Could you check a few things on this model? Use its own coordinates, in mm. A direction names the side the tool comes from. Give positions to 0.01 mm unless a question says otherwise; leave off trailing zeros. Loops run counter-clockwise (first coordinate to the right, second up) from the corner with the lowest first, then second, coordinate; pieces in that order, holes last.
1. I need wall thicknesses on line 1 along Z through (x, y) = (-50.8, -2.55); line 2 along X through (y, z) = (69, 25); line 3 along Z through (x, y) = (-10, 49). Which ranges of each line are inside material? Lowest first, please.
2. Imagine slicing it at B-B (z = 0). Count the separate pieces of the cut face and the enclosed holes in it, plus the area to 3 significant figures.
3. For P1, Ø4, axis at x = 20, y = 60.5, coming from the -Z side; P2, Ø9, axis at x = -76.2, z = -68.26, coming from the +Y side; P3, Ø1, axis at x = -65, y = 20.5, coming from the +Z side, each with a flat end and sliding along its axis, tell me the tip position at first contact or that it passes through.
4. Thinking about a two-plate mould opening in Z: for faces 4 (the flat face through (-39, 74.676, 1)), 5 (the flat face through (-39, -3, -77.66)), 6 (the cylindrical face through (-88.63, 76.25, -7.94)), which applies, +Z half, -Z half, draft (parallel to the pull), parting line (faces both ways), or undercut?
5. Imagine slicing it at A-A (y = 13.5). List the corners of the cut face in (x, z) for me.
6. For faces 1 (the flat face through (-39, 0, -67)), 2 (the flat face through (-119.15, 28, -1)), 3 (the flat face through (6, 65.024, 17)), which set-ups out of +Z, -Z, +X, -X, +Y, -Y let a thin tool reach every point of the face, with its end or its side?
```python
from build123d import *

# Parameters (mm, degrees)
BOSS_EXTRUDE1_DEPTH        = 44.45
BOSS_EXTRUDE1_DEPTH_BACK   = 120.65
SKETCH5_W                  = 99.125
SKETCH5_H                  = 72.176
BOSS_EXTRUDE2_DEPTH        = 1.5
CUT_EXTRUDE1_DEPTH         = 101.6
SKETCH12_R                 = 29
BOSS_EXTRUDE3_DEPTH        = 4.1
CHAMFER1_SIZE              = 4.1
SKETCH10_R                 = 2.05
CUT_EXTRUDE2_DEPTH         = 164.686388977
BOSS_EXTRUDE4_START        = -8.5
SKETCH17_R                 = 19.05
BOSS_EXTRUDE4_DEPTH        = 9.652
SKETCH13_R                 = 17.4625
CUT_EXTRUDE4_DEPTH         = 164.686388977
CHAMFER3_SIZE              = 1
LPATTERN1_COUNT            = 2
LPATTERN1_PITCH            = 82.55
CHAMFER1_OF_LPATTERN1_SIZE = 4.1
SKETCH14_R                 = 5
CUT_EXTRUDE5_DEPTH         = 164.686388977
SKETCH15_R                 = 10
CUT_EXTRUDE6_DEPTH         = 4.1
FILLET1_R                  = 1.27
FILLET3_R                  = 5
CHAMFER4_SIZE              = 1
CHAMFER5_SIZE              = 3
CHAMFER5_SIZE2             = 2.517298894


# Some blends are built 0.0001 mm under size
with BuildPart() as part:
    # Sketch2 → Boss-Extrude1 (new, two sides: drawn at the far end of the back side and taken through both)
    with BuildSketch(Plane(origin=(0, 0, 0), x_dir=(0, 0, -1), z_dir=(1, 0, 0)).offset(-BOSS_EXTRUDE1_DEPTH_BACK)):
        Polygon((-77.6605, 0), (-55.5625, 0), (-55.5625, 74.676), (55.5625, 74.676), (55.5625, 0), (77.6605, 0), (77.6605, -6), (49.5625, -6), (49.5625, 66.176), (-49.5625, 66.176), (-49.5625, -6), (-77.6605, -6), align=None)
    extrude(amount=BOSS_EXTRUDE1_DEPTH + BOSS_EXTRUDE1_DEPTH_BACK)

    # Sketch5 → Boss-Extrude2 (add)
    with BuildSketch(Plane.ZY.offset(120.65)):
        with Locations((0, 30.088)):
            Rectangle(SKETCH5_W, SKETCH5_H)
    extrude(amount=-BOSS_EXTRUDE2_DEPTH)

    # Sketch4 → Cut-Extrude1 (cut)
    with BuildSketch(Plane(origin=(0, 0, 0), x_dir=(1, 0, 0), z_dir=(0, 1, 0))):
        with BuildLine():
            Line((-98.85, 68.2625), (-98.85, 71.4375))
            ThreePointArc((-98.85, 71.4375), (-102.432865533, 74.058346238), (-103.845516366, 69.85))
            ThreePointArc((-103.845516366, 69.85), (-102.432865533, 65.641653762), (-98.85, 68.2625))
        make_face()
        with BuildLine():
            Line((-73.45, 68.2625), (-73.45, 71.4375))
            ThreePointArc((-73.45, 71.4375), (-77.032865533, 74.058346238), (-78.445516366, 69.85))
            ThreePointArc((-78.445516366, 69.85), (-77.032865533, 65.641653762), (-73.45, 68.2625))
        make_face()
        with BuildLine():
            Line((-48.05, 68.2625), (-48.05, 71.4375))
            ThreePointArc((-48.05, 71.4375), (-51.632865533, 74.058346238), (-53.045516366, 69.85))
            ThreePointArc((-53.045516366, 69.85), (-51.632865533, 65.641653762), (-48.05, 68.2625))
        make_face()
        with BuildLine():
            Line((-22.65, 68.2625), (-22.65, 71.4375))
            ThreePointArc((-22.65, 71.4375), (-26.232865533, 74.058346238), (-27.645516366, 69.85))
            ThreePointArc((-27.645516366, 69.85), (-26.232865533, 65.641653762), (-22.65, 68.2625))
        make_face()
        with BuildLine():
            Line((2.75, 68.2625), (2.75, 71.4375))
            ThreePointArc((2.75, 71.4375), (-0.832865533, 74.058346238), (-2.245516366, 69.85))
            ThreePointArc((-2.245516366, 69.85), (-0.832865533, 65.641653762), (2.75, 68.2625))
        make_face()
        with BuildLine():
            Line((28.15, 68.2625), (28.15, 71.4375))
            ThreePointArc((28.15, 71.4375), (24.567134467, 74.058346238), (23.154483634, 69.85))
            ThreePointArc((23.154483634, 69.85), (24.567134467, 65.641653762), (28.15, 68.2625))
        make_face()
    cut_extrude1 = extrude(amount=-CUT_EXTRUDE1_DEPTH, mode=Mode.SUBTRACT)

    # Mirror1: Cut-Extrude1 across plane
    add(cut_extrude1.mirror(Plane.XY), mode=Mode.SUBTRACT)

    # Sketch12 → Boss-Extrude3 (add)
    with BuildSketch(Plane(origin=(0, 74.676, 0), x_dir=(1, 0, 0), z_dir=(0, 1, 0))):
        with Locations(Location((0, 0, 0), (0, 0, 270))):
            Circle(SKETCH12_R)
    boss_extrude3 = extrude(amount=BOSS_EXTRUDE3_DEPTH)

    # Chamfer1
    chamfer1_edges = [part.edges().sort_by_distance(p)[0] for p in [
        (0, 74.676, -29),
    ]]
    chamfer(chamfer1_edges, length=CHAMFER1_SIZE - 0.0001)  # a hair under: the kernel refuses the full size

    # Sketch10 → Cut-Extrude2 (cut, symmetric)
    with BuildSketch(Plane(origin=(0, 0, 0), x_dir=(1, 0, 0), z_dir=(0, 1, 0))):
        with Locations(Location((17.960512242, 17.960512242, 0), (0, 0, 270))):
            Circle(SKETCH10_R)
        with Locations(Location((25.4, 0, 0), (0, 0, 270))):
            Circle(SKETCH10_R)
        with Locations(Location((17.960512242, -17.960512242, 0), (0, 0, 270))):
            Circle(SKETCH10_R)
        with Locations(Location((0, -25.4, 0), (0, 0, 270))):
            Circle(SKETCH10_R)
        with Locations(Location((-17.960512242, -17.960512242, 0), (0, 0, 270))):
            Circle(SKETCH10_R)
        with Locations(Location((-25.4, 0, 0), (0, 0, 270))):
            Circle(SKETCH10_R)
        with Locations(Location((-17.960512242, 17.960512242, 0), (0, 0, 270))):
            Circle(SKETCH10_R)
        with Locations(Location((0, 25.4, 0), (0, 0, 270))):
            Circle(SKETCH10_R)
    cut_extrude2 = extrude(amount=CUT_EXTRUDE2_DEPTH, both=True, mode=Mode.SUBTRACT)

    # Sketch17 → Boss-Extrude4 (add)
    with BuildSketch(Plane.XZ.offset(-66.176).offset(BOSS_EXTRUDE4_START)):
        with Locations(Location((0, 0, 0), (0, 0, 90))):
            Circle(SKETCH17_R)
    extrude(amount=BOSS_EXTRUDE4_DEPTH)

    # Sketch13 → Cut-Extrude4 (cut, through all)
    with BuildSketch(Plane(origin=(0, 0, 0), x_dir=(1, 0, 0), z_dir=(0, 1, 0))):
        with Locations(Location((0, 0, 0), (0, 0, 90))):
            Circle(SKETCH13_R)
    extrude(amount=CUT_EXTRUDE4_DEPTH, mode=Mode.SUBTRACT)

    # Chamfer3
    chamfer3_edges = [part.edges().sort_by_distance(p)[0] for p in [
        (0, 66.176, -19.05),
    ]]
    chamfer(chamfer3_edges, length=CHAMFER3_SIZE)

    # LPattern1: Boss-Extrude3, Cut-Extrude2 ×2
    with Locations(*[(-i * LPATTERN1_PITCH, 0, 0) for i in range(1, LPATTERN1_COUNT)]):
        add(boss_extrude3)
        add(cut_extrude2, mode=Mode.SUBTRACT)

    # Chamfer1 of LPattern1
    chamfer1_of_lpattern1_edges = [part.edges().sort_by_distance(p)[0] for p in [
        (-82.55, 74.676, -29),
    ]]
    chamfer(chamfer1_of_lpattern1_edges, length=CHAMFER1_OF_LPATTERN1_SIZE - 0.0001)  # a hair under: the kernel refuses the full size

    # Sketch14 → Cut-Extrude5 (cut, through all)
    with BuildSketch(Plane(origin=(0, 0, 0), x_dir=(1, 0, 0), z_dir=(0, 1, 0))):
        with Locations(Location((-82.55, 0, 0), (0, 0, 270))):
            Circle(SKETCH14_R)
    extrude(amount=CUT_EXTRUDE5_DEPTH, mode=Mode.SUBTRACT)

    # Sketch15 → Cut-Extrude6 (cut)
    with BuildSketch(Plane(origin=(0, 78.776, 0), x_dir=(1, 0, 0), z_dir=(0, 1, 0))):
        with Locations(Location((-82.55, 0, 0), (0, 0, 270))):
            Circle(SKETCH15_R)
    extrude(amount=-CUT_EXTRUDE6_DEPTH, mode=Mode.SUBTRACT)

    # Fillet1
    fillet1_edges = [part.edges().sort_by_distance(p)[0] for p in [
        (-38.1, 0, -55.5625),
        (-38.1, 74.676, -55.5625),
        (-38.1, 74.676, 55.5625),
        (-38.1, 0, 55.5625),
        (-37.35, -6, 49.5625),
        (-37.35, -6, -49.5625),
    ]]
    fillet(fillet1_edges, radius=FILLET1_R)

    # Fillet3
    # the kernel refuses this fillet: 5 mm, written as the material it adds along each edge
    with BuildSketch(Plane(origin=(-114.15, 61.176, 44.5625), x_dir=(0, 1, 0), z_dir=(-1, 0, 0))) as fillet3_piece_1_section:
        Polygon((0, 0), (FILLET3_R * 1.02, 0), (FILLET3_R * 1.02, -FILLET3_R * 1.02), (0, -FILLET3_R * 1.02), align=None)
    fillet3_piece_1 = extrude(amount=FILLET3_R * 1.02, mode=Mode.PRIVATE)
    fillet3_piece_1 = fillet3_piece_1 - Plane(origin=(-114.15, 61.176, 44.5625), x_dir=(0, -0.7071067811865475, -0.7071067811865475), z_dir=(-1, 0, 0)) * Sphere(FILLET3_R, mode=Mode.PRIVATE)
    add(fillet3_piece_1)
    with BuildSketch(Plane(origin=(-114.15, 61.176, -44.5625), x_dir=(-1, 0, 0), z_dir=(0, 1, 0))) as fillet3_piece_2_section:
        Polygon((0, 0), (FILLET3_R * 1.02, 0), (FILLET3_R * 1.02, -FILLET3_R * 1.02), (0, -FILLET3_R * 1.02), align=None)
    fillet3_piece_2 = extrude(amount=FILLET3_R * 1.02, mode=Mode.PRIVATE)
    fillet3_piece_2 = fillet3_piece_2 - Plane(origin=(-114.15, 61.176, -44.5625), x_dir=(0.7071067811865475, 0, 0.7071067811865475), z_dir=(0, 1, 0)) * Sphere(FILLET3_R, mode=Mode.PRIVATE)
    add(fillet3_piece_2)
    with BuildSketch(Plane(origin=(-119.15, -4.73, 49.5625), x_dir=(1, 0, 0), z_dir=(0, 1, 0))) as fillet3_piece_3:
        with BuildLine():
            CenterArc((FILLET3_R, FILLET3_R), FILLET3_R, 180, 90)
            Line((0, FILLET3_R), (0, 0))
            Line((0, 0), (FILLET3_R, 0))
        make_face()
    extrude(amount=65.906)
    with BuildSketch(Plane(origin=(-119.15, -4.73, -50.8325), x_dir=(0, 0.006283143965557515, 0.9999802608561371), z_dir=(0, -0.9999802608561371, 0.006283143965557515))) as fillet3_piece_4_section:
        with BuildLine():
            CenterArc((-1.27 - FILLET3_R, -FILLET3_R), FILLET3_R, 0, 90)
            Line((-1.27 - FILLET3_R, 0), (-1.27, 0))
            Line((-1.27, 0), (-1.27, -FILLET3_R))
        make_face()
    fillet3_piece_4 = revolve(axis=Axis((-119.15, -4.73, -50.8325), (-1, 0, 0)), revolution_arc=359.64, mode=Mode.PRIVATE)
    fillet3_piece_4 = split(fillet3_piece_4, bisect_by=Plane(origin=(-117.187917089, -6, -49.859640049), z_dir=(0, 1, 0)), keep=Keep.TOP, mode=Mode.PRIVATE)
    add(fillet3_piece_4)
    with BuildSketch(Plane(origin=(-119.15, -4.73, 50.8325), x_dir=(0, 0.006283143965559613, -0.9999802608561371), z_dir=(0, -0.9999802608561371, -0.006283143965559613))) as fillet3_piece_5_section:
        with BuildLine():
            CenterArc((-1.27 - FILLET3_R, FILLET3_R), FILLET3_R, 270, 90)
            Line((-1.27 - FILLET3_R, 0), (-1.27, 0))
            Line((-1.27, 0), (-1.27, FILLET3_R))
        make_face()
    fillet3_piece_5 = revolve(axis=Axis((-119.15, -4.73, 50.8325), (1, 0, 0)), revolution_arc=359.64, mode=Mode.PRIVATE)
    fillet3_piece_5 = split(fillet3_piece_5, bisect_by=Plane(origin=(-117.187917089, -6, 49.85964009), z_dir=(0, 1, 0)), keep=Keep.TOP, mode=Mode.PRIVATE)
    add(fillet3_piece_5)
    with BuildSketch(Plane(origin=(44.45, 66.176, 49.5625), x_dir=(0, 0, -1), z_dir=(-1, 0, 0))) as fillet3_piece_6:
        with BuildLine():
            CenterArc((FILLET3_R, FILLET3_R), FILLET3_R, 180, 90)
            Line((0, FILLET3_R), (0, 0))
            Line((0, 0), (FILLET3_R, 0))
        make_face()
    extrude(amount=158.6)
    with BuildSketch(Plane(origin=(44.45, 66.176, -49.5625), x_dir=(0, 0, 1), z_dir=(-1, 0, 0))) as fillet3_piece_7:
        with BuildLine():
            CenterArc((FILLET3_R, -FILLET3_R), FILLET3_R, 90, 90)
            Line((0, -FILLET3_R), (0, 0))
            Line((0, 0), (FILLET3_R, 0))
        make_face()
    extrude(amount=158.6)
    with BuildSketch(Plane(origin=(-119.15, 61.176, -49.5625), x_dir=(0, 0, 1), z_dir=(0, -1, 0))) as fillet3_piece_8:
        with BuildLine():
            CenterArc((FILLET3_R, -FILLET3_R), FILLET3_R, 90, 90)
            Line((0, -FILLET3_R), (0, 0))
            Line((0, 0), (FILLET3_R, 0))
        make_face()
    extrude(amount=65.906)
    with BuildSketch(Plane(origin=(-119.15, 66.176, 44.5625), x_dir=(1, 0, 0), z_dir=(0, 0, -1))) as fillet3_piece_9:
        with BuildLine():
            CenterArc((FILLET3_R, FILLET3_R), FILLET3_R, 180, 90)
            Line((0, FILLET3_R), (0, 0))
            Line((0, 0), (FILLET3_R, 0))
        make_face()
    extrude(amount=89.125)
    # the kernel refuses this fillet: 5 mm, written as the material it takes off along each edge
    with BuildSketch(Plane(origin=(-120.65, 12.5, -77.6605), x_dir=(0, 0, 1), z_dir=(0, -1, 0)), Plane(origin=(-120.65, -18.5, 77.6605), x_dir=(0, 0, -1), z_dir=(0, 1, 0))) as fillet3_2_piece_1:
        with BuildLine():
            CenterArc((FILLET3_R, -FILLET3_R), FILLET3_R, 90, 90)
            Line((0, -FILLET3_R), (0, 0))
            Line((0, 0), (FILLET3_R, 0))
        make_face()
    extrude(amount=31, mode=Mode.SUBTRACT)
    with BuildSketch(Plane(origin=(44.45, -18.5, 77.6605), x_dir=(0, 0, -1), z_dir=(0, 1, 0)), Plane(origin=(44.45, 12.5, -77.6605), x_dir=(0, 0, 1), z_dir=(0, -1, 0))) as fillet3_2_piece_2:
        with BuildLine():
            CenterArc((FILLET3_R, FILLET3_R), FILLET3_R, 180, 90)
            Line((0, FILLET3_R), (0, 0))
            Line((0, 0), (FILLET3_R, 0))
        make_face()
    extrude(amount=31, mode=Mode.SUBTRACT)

    # Chamfer4
    chamfer4_edges = [part.edges().sort_by_distance(p)[0] for p in [
        (0, 78.776, 17.4625),
        (-82.55, 66.176, -5),
        (-82.55, 74.676, -5),
        (-82.55, 78.776, -10),
    ]]
    chamfer(chamfer4_edges, length=CHAMFER4_SIZE)

    # Sketch19 → Revolve1 (revolve)
    with BuildSketch(Plane(origin=(0, 0, 0), x_dir=(0, 0, -1), z_dir=(1, 0, 0)), mode=Mode.PRIVATE) as revolve1_sk:
        Polygon((30, 66.176), (30, 62.121804358), (40, 62.821072478), (40, 66.176), align=None)
    revolve(revolve1_sk.sketch.rotate(Axis((0, 83.1148, 0), (0, -1, 0)), 180), axis=Axis((0, 83.1148, 0), (0, -1, 0)))

    # Chamfer5
    chamfer5_edges = [part.edges().sort_by_distance(p)[0] for p in [
        (0, 66.176, -40),
    ]]
    chamfer5_side = [part.faces().sort_by_distance(p)[0] for p in [
        (0, 64.498536239, -40),
    ]]
    chamfer(chamfer5_edges, length=CHAMFER5_SIZE, length2=CHAMFER5_SIZE2, reference=chamfer5_side[0])


solid = part.part
```
Derived:
1. line 1: z = -77.66 to -74.19, -65.51 to -49.56, 49.56 to 65.51, 74.19 to 77.66
1. line 2: x = -120.65 to -84.56, -80.54 to -2.01, 2.01 to 44.45
1. line 3: z = -55.56 to -49.56, 49.56 to 55.56
2. separate pieces: 7
2. enclosed holes: 0
2. area: 1,290 mm2
3. P1: stops at z = -55.56
3. P2: stops at y = 0
3. P3: stops at z = 55.56
4. face 4: draft
4. face 5: -Z half
4. face 6: undercut
5. outline: (-120.65, -55.56) - (44.45, -55.56) - (44.45, -49.56) - (-114.15, -49.56) arc R5 cw to (-119.15, -44.56) - (-119.15, 44.56) arc R5 cw to (-114.15, 49.56) - (44.45, 49.56) - (44.45, 55.56) - (-120.65, 55.56) - close
6. face 1: -Z, +X, -X, +Y
6. face 2: +X, -Y
6. face 3: -Y
